from build123d import *

# Parameters (mm, degrees)
SKETCH1_R           = 3.8
BOSS_EXTRUDE1_DEPTH = 2.2
SKETCH2_R           = 2
BOSS_EXTRUDE2_DEPTH = 16
CHAMFER1_SIZE       = 0.3
CUT_EXTRUDE1_DEPTH  = 2
FILLET1_R           = 1.8


with BuildPart() as part:
    # Sketch1 → Boss-Extrude1 (new body)
    with BuildSketch(Plane.XY):
        Circle(SKETCH1_R)
    extrude(amount=BOSS_EXTRUDE1_DEPTH)

    # Sketch2 → Boss-Extrude2 (add)
    with BuildSketch(Plane(origin=(0, 0, 0), x_dir=(-1, 0, 0), z_dir=(0, 0, -1))):
        Circle(SKETCH2_R)
    extrude(amount=BOSS_EXTRUDE2_DEPTH)

    # Chamfer1
    chamfer1_edges = [part.edges().sort_by_distance(p)[0] for p in [
        (2, 0, -16),
    ]]
    chamfer(chamfer1_edges, length=CHAMFER1_SIZE)

    # Sketch3 → Cut-Extrude1 (cut)
    with BuildSketch(Plane.XY.offset(2.2)):
        Polygon((0, 1.443375673), (-1.25, 0.721687836), (-1.25, -0.721687836), (0, -1.443375673), (1.25, -0.721687836), (1.25, 0.721687836), align=None)
    extrude(amount=-CUT_EXTRUDE1_DEPTH, mode=Mode.SUBTRACT)

    # Fillet1
    fillet1_edges = [part.edges().sort_by_distance(p)[0] for p in [
        (-3.8, 0, 2.2),
    ]]
    fillet(fillet1_edges, radius=FILLET1_R)


solid = part.part
Work out the finished part from the listing and answer in its coordinate system (mm). A direction names the side the tool comes from. Round coordinates to 2 decimals unless told otherwise and drop trailing zeros. Write each loop counter-clockwise with the first axis right and the second up, starting at its lowest first coordinate (ties: lowest second). Pieces come first, ordered by that corner, then holes. Notation, with made-up numbers: (-21.75, 21) -> (1.25, 21) arc R25 cw to (1.25, 55) -> close; hole circle Ø2 at (-25, 28). An arc over 180 degrees is marked (long way). Answer as CSV lines item,"result". Start each with the question number.
(1) Find the intervals of material crossed by probe 1 along Y at (x, z) = (0, -7); probe 2 along Z at (x, y) = (-0.25, 0.25); probe 3 along Z at (x, y) = (3, 1.25), in increasing order.
(2) Each of these flat-tipped pins is pushed along its axis until it touches: pin 1 (1 mm diameter, centred on y = 0.5, z = -8, fed in from -X); pin 2 (3 mm diameter, centred on y = -1, z = -2, fed in from +X); pin 3 (1.6 mm diameter, centred on y = 0, z = 1.5, fed in from -X). Where does it stop, or does it pass through?
(3) A tool of negligible diameter and unlimited length cuts with its end or side. For faces 4 (the flat face through (2, -2, 0)), 5 (the flat face through (1.25, 0, 1)), from which of +Z, -Z, +X, -X, +Y, -Y can it reach the whole face along a straight path? Write none if from no direction.
(4) The part is cut by section A-A, the plane y = 0. Give the vertices of the cut face in (x, z).
(5) The part is cut by section B-B, the plane z = 1.25. Give the vertices of the cut face in (x, y).
(6) The mould has two halves that part along Y. Classify faces 1 (the flat face through (0, 0, -16)), 2 (the flat face through (-1.25, 0, 1)), 3 (the cylindrical face through (-3.796, 0.167, 0.197)): +Y half, -Y half, draft (parallel to the pull), parting line (faces both ways), or undercut.
Output values:
1,probe 1,"y = -2 to 2"
1,probe 2,"z = -16 to 0.2"
1,probe 3,"z = 0 to 1.7"
2,pin 1,"stops at x = -2"
2,pin 2,"stops at x = 2"
2,pin 3,"stops at x = -3.77"
3,face 4,"-Z"
3,face 5,"+Z"
4,outline,"(-3.8, 0) -> (-2, 0) -> (-2, -15.7) -> (-1.7, -16) -> (1.7, -16) -> (2, -15.7) -> (2, 0) -> (3.8, 0) -> (3.8, 0.4) arc R1.8 ccw to (2, 2.2) -> (1.25, 2.2) -> (1.25, 0.2) -> (-1.25, 0.2) -> (-1.25, 2.2) -> (-2, 2.2) arc R1.8 ccw to (-3.8, 0.4) -> close"
5,outline,"circle Ø7.17 at (0, 0); hole (-1.25, -0.72) -> (0, -1.44) -> (1.25, -0.72) -> (1.25, 0.72) -> (0, 1.44) -> (-1.25, 0.72) -> close"
6,face 1,"draft"
6,face 2,"undercut"
6,face 3,"parting line"
